Geometry: final body of the model. Coordinates: model frame, mm. A direction names the side the tool comes from. Round coordinates to 2 decimals unless told otherwise and drop trailing zeros. Loops run counter-clockwise (first coordinate to the right, second up) from the corner with the lowest first, then second, coordinate; pieces in that order, holes last. Notation, with made-up numbers: (68, 26.25) -> (120, 26.25) arc R23 cw to (120, 53.25) -> close; hole circle Ø1 at (19.5, 45). An arc over 180 degrees is marked (long way). Answer in a Markdown table with one row per item.
```python
from build123d import *

# Parameters (mm, degrees)
SKETCH1_W                = 100
SKETCH1_H                = 100
SKETCH1_R                = 23.682087014
BOSS_EXTRUDE1_DEPTH      = 10
SKETCH2_W                = 100
SKETCH2_H                = 24
BOSS_EXTRUDE2_DEPTH      = 20
BOSS_EXTRUDE3_DEPTH      = 20
BOSS_EXTRUDE3_DEPTH_BACK = 10
SKETCH2_3_W              = 20
SKETCH2_3_H              = 32


with BuildPart() as part:
    # Sketch1 → Boss-Extrude1 (new body)
    with BuildSketch(Plane(origin=(0, 0, 0), x_dir=(1, 0, 0), z_dir=(0, 1, 0))):
        Rectangle(SKETCH1_W, SKETCH1_H)
        with Locations(Location((0, 0, 0), (0, 0, 270))):
            Circle(SKETCH1_R, mode=Mode.SUBTRACT)
    extrude(amount=BOSS_EXTRUDE1_DEPTH)

    # Sketch2 → Boss-Extrude2 (add)
    with BuildSketch(Plane.XZ):
        with Locations((0, 38)):
            Rectangle(SKETCH2_W, SKETCH2_H)
        Polygon((77, 58), (-58, 58), (-58, 26), (-50, 26), (-50, 50), (50, 50), (50, 26), (77, 26), align=None)
        Polygon((-50, -50), (-50, -26), (-58, -26), (-58, -58), (77, -58), (77, -26), (50, -26), (50, -50), align=None)
        with Locations((0, -38)):
            Rectangle(SKETCH2_W, SKETCH2_H)
    extrude(amount=BOSS_EXTRUDE2_DEPTH)

    # Sketch2_3 → Boss-Extrude3 (add, two sides: drawn at the far end of the back side and taken through both)
    with BuildSketch(Plane.XZ.offset(-BOSS_EXTRUDE3_DEPTH_BACK)):
        with Locations((87, -42)):
            Rectangle(SKETCH2_3_W, SKETCH2_3_H)
        with Locations((87, 42)):
            Rectangle(SKETCH2_3_W, SKETCH2_3_H)
    extrude(amount=BOSS_EXTRUDE3_DEPTH + BOSS_EXTRUDE3_DEPTH_BACK)


solid = part.part
```
Item 1: Section query D-D, the plane x = 41.5. Output: boundary loops of the cut face in (y, z).
Ans:
| item | result |
|---|---|
| outline | (-20, -58) -> (0, -58) -> (0, -50) -> (10, -50) -> (10, 50) -> (0, 50) -> (0, 58) -> (-20, 58) -> (-20, 26) -> (0, 26) -> (0, -26) -> (-20, -26) -> close |
Item 2: First-contact query: P1, Ø3, axis at x = -22.5, y = 5, coming from the -Z side; P2, Ø3, axis at x = 34.5, z = 7.5, coming from the -Y side; P3, Ø4, axis at y = -1, z = -10.5, coming from the +X side. Flat tips, straight axial feed; report the tip coordinate or a pass-through.
Ans:
| item | result |
|---|---|
| P1 | z = -50 |
| P2 | y = 0 |
| P3 | x = 50 |
Item 3: Section query B-B, the plane z = 0. Output: boundary loops of the cut face in (x, y), and give its area (3 significant figures).
Ans:
| item | result |
|---|---|
| outline | (-50, 0) -> (-23.68, 0) -> (-23.68, 10) -> (-50, 10) -> close; (23.68, 0) -> (50, 0) -> (50, 10) -> (23.68, 10) -> close |
| area | 526 mm2 |
Item 4: Mould query, pull axis X, two halves, no side actions, for faces 1 (the flat face through (50, 5, 1)), 2 (the flat face through (-23, 10, -12)), 3 (the flat face through (-58, -10, 42)), 4 (the flat face through (24, 0, -52)). Classes: released by +X, released by -X, zero draft, split by the parting line, or undercut.
Ans:
| item | result |
|---|---|
| face 1 | undercut |
| face 2 | zero draft |
| face 3 | released by -X |
| face 4 | undercut |
Item 5: Set-up query: faces 5 (the flat face through (77, 5, 42)), 6 (the flat face through (-23, 0, -12)), 7 (the flat face through (-1, 5, 50)), 8 (the flat face through (-1, 5, -50)). Return all of +Z, -Z, +X, -X, +Y, -Y with unobstructed straight access to the full face (end or side cutting, diameter ignored); none if empty.
Ans:
| item | result |
|---|---|
| face 5 | +Z, -Z, +Y |
| face 6 | +X, -X, -Y |
| face 7 | +Z, -X, +Y |
| face 8 | -Z, -X, +Y |
Item 6: Section query A-A, the plane x = 0. Output: boundary loops of the cut face in (y, z), and give its area (3 significant figures).
Ans:
| item | result |
|---|---|
| outline | (-20, -58) -> (0, -58) -> (0, -50) -> (10, -50) -> (10, -23.68) -> (0, -23.68) -> (0, -26) -> (-20, -26) -> close; (-20, 26) -> (0, 26) -> (0, 23.68) -> (10, 23.68) -> (10, 50) -> (0, 50) -> (0, 58) -> (-20, 58) -> close |
| area | 1,810 mm2 |
Item 7: Section query C-C, the plane y = -4. Output: boundary loops of the cut face in (x, z), and give its area (3 significant figures).
Ans:
| item | result |
|---|---|
| outline | (-58, -58) -> (97, -58) -> (97, -26) -> (-58, -26) -> close; (-58, 26) -> (97, 26) -> (97, 58) -> (-58, 58) -> close |
| area | 9,920 mm2 |
Item 8: Ray query, L1, parallel to X at y = 6, z = 0; L2, parallel to Z at x = -38, y = -8.5; L3, parallel to Y at x = 62, z = -36. Return the intervals inside material, ascending.
Ans:
| item | result |
|---|---|
| L1 | -50 to -23.68, 23.68 to 50 |
| L2 | -58 to -26, 26 to 58 |
| L3 | -20 to 0 |
